Autodesk Inventor part; units mm, degrees
ref_plane "YZ Plane" through (0, 0, 0) normal (1, 0, 0) x (0, 1, 0)
ref_plane "XZ Plane" through (0, 0, 0) normal (0, 1, 0) x (-1, 0, 0)
ref_plane "XY Plane" through (0, 0, 0) normal (0, 0, 1) x (1, 0, 0)
sketch "Skizze1" plane through (0, 0, 0) normal (0, 1, 0) x (-1, 0, 0)
  line L0 (0, 0) -> (17, 0)
  line L1 (17, 0) -> (17, -40)
  line L2 (17, -40) -> (0, -40)
  line L3 (0, -40) -> (0, 0)
  dimension "d0" = 17
  dimension "d1" = 40
extrude "Extrusion1" add sketch "Skizze1" along normal blind 5
sketch "Skizze2" plane through (0, 5, 0) normal (0, 1, 0) x (1, 0, 0)
  line L0 (-17, 0) -> (0, 0)
  line L1 (0, 0) -> (0, 40)
  line L2 (-17, 0) -> (0, 0)
  line L3 (0, 0) -> (0, 10)
  line L4 (0, 10) -> (-17, 10)
  line L5 (-17, 10) -> (-17, 0)
  dimension "d4" = 10
extrude "Extrusion2" add sketch "Skizze2" along normal blind 11
sketch "Skizze3" plane through (0, 16, 0) normal (0, 1, 0) x (1, 0, 0)
  line L0 (-17, 0) -> (0, 0)
  line L1 (0, 0) -> (0, 40)
  line L2 (-17, 0) -> (0, 0)
  line L3 (0, 0) -> (0, 40)
  line L4 (0, 40) -> (-17, 40)
  line L5 (-17, 40) -> (-17, 0)
  dimension "d7" = 17
  dimension "d8" = 40
extrude "Extrusion3" add sketch "Skizze3" along normal blind 5
sketch "Skizze4" plane through (0, 21, 0) normal (0, 1, 0) x (1, 0, 0)
  line L0 (0, 10) -> (0, 40)
  line L1 (0, 40) -> (-8.5, 40)
  line L2 (-8.5, 40) -> (-8.5, 25)
  line L3 (-8.5, 25) -> (0, 25)
  line L4 (0, 25) -> (0, 40)
  circle A0 centre (-8.5, 25) radius 4.5
  point P0 (0, 0)
  dimension "d11" = 8.5
  dimension "d12" = 15
  dimension "d13" = 9
extrude "Extrusion4" cut sketch "Skizze4" against normal blind 21 contours A0 L2 L3 | L3 L2 A0
sketch "Skizze5" plane through (0, 21, 0) normal (0, 1, 0) x (1, 0, 0)
  circle A0 centre (-8.5, 25) radius 4.5
  line L0 (-8.5, 25) -> (0, 25)
  line L1 (0, 0) -> (0, 40)
  line L2 (0, 25) -> (-2, 25)
  line L3 (-2, 25) -> (-3.25, 25)
  line L4 (-3.25, 25) -> (-3.25, 27.55)
  line L5 (-3.25, 27.55) -> (-0.75, 27.55)
  line L6 (-0.75, 27.55) -> (-0.75, 22.45)
  line L7 (-0.75, 22.45) -> (-3.25, 22.45)
  line L8 (-3.25, 22.45) -> (-3.25, 25)
  dimension "d16" = 2
  dimension "d17" = 1.25
  dimension "d18" = 2.55
  dimension "d19" = 2.5
  dimension "d20" = 5.1
extrude "Extrusion5" cut sketch "Skizze5" against normal blind 5 contours L4 L5 L6 L0 | L0 L6 L7 L8
sketch "Skizze6" plane through (0, 5, 0) normal (0, 1, 0) x (1, 0, 0)
  point P0 (0, 0)
sketch "Skizze7" plane through (0, 21, 0) normal (0, 1, 0) x (1, 0, 0)
  point P0 (0, 0)
sketch "Skizze8" plane through (0, 0, 0) normal (1, 0, 0) x (0, 0, -1)
  line L0 (40, 16) -> (40, 21)
  line L1 (40, 20.3408) -> (25, 20.3408)
  line L2 (40, 20.3408) -> (55, 20.3408) construction
  line L3 (25, 20.3408) -> (25, 21)
  line L4 (27.55, 21) -> (22.45, 21)
  line L5 (25, 21) -> (25, 18.5)
  circle A0 centre (25, 18.5) radius 1.5
  point P0 (0, 0)
  dimension "d23" = 15
  dimension "d24" = 180
  dimension "d25" = 2.5
  dimension "d26" = 3
extrude "Extrusion6" cut sketch "Skizze8" against normal blind 10
sketch "Skizze9" plane through (0, 21, 0) normal (0, 1, 0) x (1, 0, 0)
  point P0 (0, 0)
sketch "Skizze10" plane through (0, 21, 0) normal (0, 1, 0) x (1, 0, 0)
  point P0 (0, 0)
sketch "Skizze11" plane through (0, 5, 0) normal (0, 1, 0) x (1, 0, 0)
  point P0 (0, 0)
sketch "Skizze12" plane through (-17, 0, -40) normal (-1, 0, 0) x (0, 0, 1)
  line L0 (40, 21) -> (0, 21)
  line L1 (40, 0) -> (0, 0)
  line L2 (40, 21) -> (30, 21)
  line L3 (30, 0) -> (40, 0)
  line L4 (40, 0) -> (40, 21)
  line L5 (30, 16) -> (0, 16)
  line L6 (30, 21) -> (0, 21)
  line L7 (0, 21) -> (0, 16)
  line L8 (0, 16) -> (30, 16)
  line L9 (30, 5) -> (30, 16)
  line L10 (30, 5) -> (0, 5)
  line L11 (0, 5) -> (0, 0)
  line L12 (0, 0) -> (30, 0)
  line L13 (30, 16) -> (30, 5)
  dimension "d29" = 10
extrude "Extrusion7" add sketch "Skizze12" along normal blind 2.5
sketch "Skizze13" plane through (0, 0, 0) normal (1, 0, 0) x (0, 0, -1)
  line L0 (0, 0) -> (40, 0)
  line L1 (10, 5) -> (40, 5)
  line L2 (40, 0) -> (10, 0)
  line L3 (10, 5) -> (40, 5)
  line L4 (40, 5) -> (40, 0)
  line L5 (0, 0) -> (0, 21)
  line L6 (10, 0) -> (0, 0)
  line L7 (0, 0) -> (0, 21)
  line L8 (0, 21) -> (10, 21)
  line L9 (10, 16) -> (40, 16)
  line L10 (40, 16) -> (10, 16)
  line L11 (10, 21) -> (40, 21)
  line L12 (40, 21) -> (40, 16)
  line L13 (10, 5) -> (10, 16)
  line L14 (10, 5) -> (10, 16)
  circle A0 centre (25, 18.5) radius 1.5
  circle A1 centre (25, 18.5) radius 1.5
  dimension "d32" = 3
extrude "Extrusion8" add sketch "Skizze13" along normal blind 2.5
sketch "Skizze14" plane through (0, 21, 0) normal (0, 1, 0) x (1, 0, 0)
  line L0 (-0.75, 27.55) -> (-3.25, 27.55)
  line L1 (-3.25, 22.45) -> (-3.25, 27.55)
  line L2 (-0.75, 27.55) -> (-3.25, 27.55)
  line L3 (-3.25, 27.55) -> (-3.25, 22.45)
  line L4 (-3.25, 22.45) -> (-0.75, 22.45)
  line L5 (-0.75, 22.45) -> (-0.75, 27.55)
  point P0 (0, 0)
extrude "Extrusion9" add sketch "Skizze14" against normal blind 5
sketch "Skizze15" plane through (0, 21, 0) normal (0, 1, 0) x (1, 0, 0)
  circle A0 centre (-8.5, 25) radius 4.5
  line L0 (-8.5, 25) -> (2.5, 25)
  line L1 (2.5, 26.5) -> (2.5, 23.5)
  line L2 (2.5, 25) -> (-4, 25)
  line L3 (2.5, 25) -> (-0.75, 25)
  line L4 (-0.75, 25) -> (-2, 25)
  line L5 (-2, 25) -> (-2, 22.45)
  line L6 (-2, 22.45) -> (0.5, 22.45)
  line L7 (0.5, 22.45) -> (0.5, 27.55)
  line L8 (0.5, 27.55) -> (-2, 27.55)
  line L9 (0.5, 27.55) -> (3, 27.55) construction
  line L10 (-2, 27.55) -> (-2, 25)
  point P0 (0, 0)
  dimension "d37" = 3.25
  dimension "d38" = 1.25
  dimension "d39" = 2.55
  dimension "d40" = 90
  dimension "d41" = 2.5
  dimension "d42" = 90
  dimension "d43" = 5.1
  dimension "d44" = 90
  dimension "d45" = 2.5
  dimension "d46" = 180
sketch "Skizze16" plane through (0, 21, 0) normal (0, 1, 0) x (1, 0, 0)
  point P0 (0, 0)
extrude "Extrusion10" cut sketch "Skizze15" against normal blind 5 contours L10 L8 L7 L0 | L0 L7 L6 L5
sketch "Skizze17" plane through (2.5, 0, 0) normal (1, 0, 0) x (0, 0, -1)
  circle A0 centre (25, 18.5) radius 1.5
  circle A1 centre (25, 18.5) radius 1.5
  point P0 (0, 0)
  dimension "d49" = 3
sketch "Skizze18" plane through (-3.25, 18.5, -25) normal (-1, 0, 0) x (0, 0, 1)
  circle A0 centre (0, 0) radius 1.5
  point P0 (25, -18.5)
  dimension "d50" = 3
extrude "Extrusion11" cut sketch "Skizze18" against normal blind 8
sketch "Skizze19" plane through (-19.5, 0, 0) normal (0, 0, 1) x (1, 0, 0)
  line L0 (22, 0) -> (0, 0)
  line L1 (0, 21) -> (0, 16)
  line L2 (22, 0) -> (0, 0)
  line L3 (0, 0) -> (0, 21)
  line L4 (0, 21) -> (22, 21)
  line L5 (22, 21) -> (22, 0)
  point P0 (19.5, 0)
extrude "Extrusion12" add sketch "Skizze19" along normal blind 5
sketch "Skizze20" plane through (-19.5, 5, -10) normal (0, 0, -1) x (-1, 0, 0)
  line L0 (0, 11) -> (0, 0)
  line L1 (0, 11) -> (-22, 11)
  line L2 (0, 0) -> (-22, 0)
  line L3 (-22, 0) -> (-22, 11)
  line L4 (-22, 11) -> (0, 11)
  line L5 (0, 11) -> (0, 0)
  point P0 (-19.5, -5)
extrude "Extrusion13" cut sketch "Skizze20" against normal blind 5
sketch "Skizze21" plane through (-19.5, 0, -40) normal (-1, 0, 0) x (0, 0, 1)
  line L0 (0, 0) -> (45, 0)
  line L1 (0, 5) -> (45, 5)
  line L2 (45, 5) -> (45, 0)
  line L3 (45, 0) -> (0, 0)
  line L4 (0, 0) -> (0, 5)
  point P0 (40, 0)
extrude "Extrusion14" add sketch "Skizze21" along normal blind 13.5
sketch "Skizze22" plane through (2.5, 0, 0) normal (1, 0, 0) x (0, 0, -1)
  line L0 (40, 0) -> (-5, 0)
  line L1 (40, 5) -> (5, 5)
  line L2 (-5, 0) -> (40, 0)
  line L3 (40, 0) -> (40, 5)
  line L4 (40, 5) -> (-5, 5)
  line L5 (-5, 5) -> (-5, 0)
  point P0 (0, 0)
extrude "Extrusion15" add sketch "Skizze22" along normal blind 13.5
sketch "Skizze23" plane through (0, 5, 0) normal (0, 1, 0) x (1, 0, 0)
  line L0 (16, 40) -> (10, 40)
  line L1 (10, 40) -> (10, 34)
  line L2 (10, 34) -> (16, 34)
  line L3 (16, 34) -> (16, 40)
  circle A0 centre (10, 34) radius 1.5
  point P0 (0, 0)
  dimension "d61" = 6
  dimension "d62" = 6
  dimension "d63" = 3
extrude "Extrusion16" cut sketch "Skizze23" against normal blind 13.5 contours A0 L2 L1 | L1 L2 A0
sketch "Skizze24" plane through (0, 5, 0) normal (0, 1, 0) x (1, 0, 0)
  line L0 (16, -5) -> (16, 40)
  line L1 (16, -5) -> (10, -5)
  line L2 (10, -5) -> (10, 1)
  line L3 (10, 1) -> (16, 1)
  line L4 (16, 1) -> (16, -5)
  circle A0 centre (10, 1) radius 1.5
  point P0 (0, 0)
  dimension "d66" = 6
  dimension "d67" = 6
  dimension "d68" = 3
extrude "Extrusion17" cut sketch "Skizze24" against normal blind 13.5 contours A0 L2 L3 | L3 L2 A0
sketch "Skizze25" plane through (0, 5, 0) normal (0, 1, 0) x (1, 0, 0)
  line L0 (-33, 40) -> (-33, -5)
  line L1 (-33, 40) -> (-27, 40)
  line L2 (-27, 40) -> (-27, 34)
  line L3 (-27, 34) -> (-33, 34)
  line L4 (-33, 34) -> (-33, 40)
  circle A0 centre (-27, 34) radius 1.5
  point P0 (0, 0)
  dimension "d71" = 6
  dimension "d72" = 6
  dimension "d73" = 3
extrude "Extrusion18" cut sketch "Skizze25" against normal blind 13.5 contours A0 L2 L3 | L3 L2 A0
sketch "Skizze26" plane through (0, 5, 0) normal (0, 1, 0) x (1, 0, 0)
  line L0 (16, -5) -> (-33, -5)
  line L1 (-33, -5) -> (-27, -5)
  line L2 (-27, -5) -> (-27, 1)
  line L3 (-27, 1) -> (-33, 1)
  line L4 (-33, 1) -> (-33, -5)
  circle A0 centre (-27, 1) radius 1.5
  point P0 (0, 0)
  dimension "d76" = 6
  dimension "d77" = 6
  dimension "d78" = 3
extrude "Extrusion19" cut sketch "Skizze26" against normal blind 13.5 contours A0 L3 L2 | L2 L3 A0
sketch "Skizze27" plane through (0, 5, 0) normal (0, 1, 0) x (1, 0, 0)
  line L0 (2.5, -5) -> (16, -5)
  line L1 (16, 40) -> (16, -5)
  line L2 (2.5, -5) -> (16, -5)
  line L3 (16, -5) -> (16, 40)
  line L4 (16, 40) -> (2.5, 40)
  line L5 (2.5, 40) -> (2.5, -5)
  point P0 (0, 0)
extrude "Extrusion20" cut sketch "Skizze27" against normal blind 10
sketch "Skizze28" plane through (0, 5, 0) normal (0, 1, 0) x (1, 0, 0)
  line L0 (-19.5, 5) -> (-19.5, -5)
  line L1 (-33, -5) -> (-33, 40)
  line L2 (-19.5, -5) -> (-33, -5)
  line L3 (-33, -5) -> (-33, 40)
  line L4 (-33, 40) -> (-19.5, 40)
  line L5 (-19.5, 40) -> (-19.5, -5)
  point P0 (0, 0)
extrude "Extrusion21" cut sketch "Skizze28" against normal blind 10
sketch "Skizze29" plane through (0, 0, 0) normal (0, -1, 0) x (1, 0, 0)
  line L0 (2.5, 5) -> (-19.5, 5)
  line L1 (-19.5, -40) -> (-19.5, -5)
  line L2 (2.5, 5) -> (-19.5, 5)
  line L3 (-19.5, 5) -> (-19.5, -40)
  line L4 (-19.5, -40) -> (2.5, -40)
  line L5 (2.5, -40) -> (2.5, 5)
  point P0 (0, 0)
extrude "Extrusion22" add sketch "Skizze29" along normal blind 10
sketch "Skizze30" plane through (0, 5, 0) normal (0, 1, 0) x (1, 0, 0)
  circle A0 centre (-8.5, 25) radius 4.5
  circle A1 centre (-8.5, 25) radius 4.5
  point P0 (0, 0)
  dimension "d87" = 9
extrude "Extrusion23" add sketch "Skizze30" against normal blind 5
extrude "Extrusion24" cut sketch "Skizze30" against normal blind 15
sketch "Skizze31" plane through (2.5, 5, -40) normal (0, 0, -1) x (-1, 0, 0)
  point P0 (2.5, -5)
sketch "Skizze32" plane through (2.5, 0, 0) normal (1, 0, 0) x (0, 0, -1)
  line L0 (-5, -10) -> (-5, 21)
  line L1 (-5, -10) -> (40, -10)
  line L2 (40, -10) -> (40, -5)
  line L3 (40, -5) -> (-5, -5)
  line L4 (-5, -5) -> (-5, -10)
  point P0 (0, 0)
  dimension "d92" = 45
  dimension "d93" = 5
extrude "Extrusion25" add sketch "Skizze32" along normal blind 13.5
sketch "Skizze33" plane through (-19.5, 0, -40) normal (-1, 0, 0) x (0, 0, 1)
  line L0 (45, -10) -> (0, -10)
  line L1 (0, -10) -> (45, -10)
  line L2 (45, -10) -> (45, -5)
  line L3 (45, -5) -> (0, -5)
  line L4 (0, -5) -> (0, -10)
  point P0 (40, 0)
  dimension "d96" = 45
  dimension "d97" = 5
extrude "Extrusion26" add sketch "Skizze33" along normal blind 13.5
sketch "Skizze34" plane through (-19.5, -5, 5) normal (0, 1, 0) x (1, 0, 0)
  line L0 (35.5, 45) -> (-13.5, 45)
  line L1 (-13.5, 45) -> (-7.5, 45)
  line L2 (-7.5, 45) -> (-7.5, 39)
  line L3 (-7.5, 39) -> (-13.5, 39)
  line L4 (-13.5, 39) -> (-13.5, 45)
  circle A0 centre (-7.5, 39) radius 1.5
  point P0 (19.5, 5)
  dimension "d100" = 6
  dimension "d101" = 6
  dimension "d102" = 3
extrude "Extrusion27" cut sketch "Skizze34" against normal blind 5 contours A0 L3 L2 | L2 L3 A0
sketch "Skizze35" plane through (-19.5, -5, 5) normal (0, 1, 0) x (1, 0, 0)
  line L0 (0, 0) -> (-13.5, 0)
  line L1 (-13.5, 0) -> (-7.5, 0)
  line L2 (-7.5, 0) -> (-7.5, 6)
  line L3 (-7.5, 6) -> (-13.5, 6)
  line L4 (-13.5, 6) -> (-13.5, 0)
  circle A0 centre (-7.5, 6) radius 1.5
  point P0 (19.5, 5)
  dimension "d105" = 6
  dimension "d106" = 6
  dimension "d107" = 3
extrude "Extrusion28" cut sketch "Skizze35" against normal blind 5 contours A0 L3 L2 | L2 L3 A0
sketch "Skizze36" plane through (2.5, -5, 5) normal (0, 1, 0) x (1, 0, 0)
  line L0 (13.5, 0) -> (13.5, 45)
  line L1 (13.5, 45) -> (7.5, 45)
  line L2 (7.5, 45) -> (7.5, 39)
  line L3 (7.5, 39) -> (13.5, 39)
  line L4 (13.5, 39) -> (13.5, 45)
  circle A0 centre (7.5, 39) radius 1.5
  point P0 (-2.5, 5)
  dimension "d110" = 6
  dimension "d111" = 6
  dimension "d112" = 3
sketch "Skizze37" plane through (2.5, -5, 5) normal (0, 1, 0) x (1, 0, 0)
  point P0 (-2.5, 5)
extrude "Extrusion29" cut sketch "Skizze36" against normal blind 5 contours A0 L2 L3 | L3 L2 A0
sketch "Skizze38" plane through (2.5, -5, 5) normal (0, 1, 0) x (1, 0, 0)
  line L0 (13.5, 0) -> (13.5, 45)
  line L1 (13.5, 0) -> (7.5, 0)
  line L2 (7.5, 0) -> (7.5, 6)
  line L3 (7.5, 6) -> (13.5, 6)
  line L4 (13.5, 6) -> (13.5, 0)
  circle A0 centre (7.5, 6) radius 1.5
  point P0 (-2.5, 5)
  dimension "d115" = 6
  dimension "d116" = 6
  dimension "d117" = 3
extrude "Extrusion30" cut sketch "Skizze38" against normal blind 5 contours A0 L2 L3 | L3 L2 A0
properties part number "HalterungRillenKugelLager"
Check sheet for the modelled part. Datum: model origin and axes. Units: mm. A direction names the side the tool comes from. Give positions to 0.01 mm unless a question says otherwise; leave off trailing zeros. Write each loop counter-clockwise with the first axis right and the second up, starting at its lowest first coordinate (ties: lowest second). Pieces come first, ordered by that corner, then holes.
Item 1: Cross-section at B-B (x = 10). Enter the section's corners in (y, z), and give its area (3 significant figures).
Item 2: Gauge pin test, flat ends, axial feed: pin 1 (5.5 mm diameter, centred on y = 19, z = -25, fed in from +X); pin 2 (4 mm diameter, centred on y = 15, z = -11.5, fed in from -X); pin 3 (1.5 mm diameter, centred on x = 11, z = -23.5, fed in from +Y). Record the tip position at first contact, or that the pin passes through.
Item 3: Cross-section at D-D (y = 18.5). Enter the section's corners in (x, z), and give its area (3 significant figures).
Item 4: Cross-section at A-A (z = -16.5). Enter the section's corners in (x, y).
Item 5: Cross-section at C-C (z = -1). Enter the section's corners in (x, y).
Item 6: Access from +Z, -Z, +X, -X, +Y, -Y to the whole of each face (thin tool, end or side, straight path). Record for faces 1 (the face through (2.5, 2, -13)), 2 (the face through (1.49, 17.49, -23.89)), 3 (the face through (0.5, 20, -24)), 4 (the face through (-9, 5, -19)).
Item 7: Scan lines: L1, parallel to Z at x = -27, y = -7; L2, parallel to X at y = -6.2, z = -1; L3, parallel to Z at x = -8.5, y = -1. Record each from-to range of solid material in increasing order.
Item 8: Draft check along X on faces 5 (the face through (-1, 19, -22.45)), 6 (the face through (-2, 20, -26)), 7 (the face through (-19.5, 2, -13)), 8 (the face through (-8, -4, -40)). Enter one of: released by +X, released by -X, zero draft, split by the parting line, or undercut.
Report:
1. outline: (-10, -40) - (-5, -40) - (-5, -35.5) - (-10, -35.5) - close; (-10, -32.5) - (-5, -32.5) - (-5, -2.5) - (-10, -2.5) - close; (-10, 0.5) - (-5, 0.5) - (-5, 5) - (-10, 5) - close
1. area: 195 mm2
2. pin 1: stops at x = 2.5
2. pin 2: stops at x = -19.5
2. pin 3: stops at y = -5
3. outline: (-19.5, -40) - (2.5, -40) - (2.5, -26.5) - (0.5, -26.5) - (0.5, -27.55) - (-2, -27.55) - (-2, -26.5) - (-4.26, -26.5) arc R4.5 cw (long way) to (-4.26, -23.5) - (-2, -23.5) - (-2, -22.45) - (0.5, -22.45) - (0.5, -23.5) - (2.5, -23.5) - (2.5, 5) - (-19.5, 5) - close
3. area: 901 mm2
4. outline: (-33, -10) - (16, -10) - (16, -5) - (2.5, -5) - (2.5, 5) - (-19.5, 5) - (-19.5, -5) - (-33, -5) - close; (-19.5, 16) - (2.5, 16) - (2.5, 21) - (-19.5, 21) - close
5. outline: (-33, -10) - (-28.5, -10) - (-28.5, -5) - (-33, -5) - close; (-25.5, -10) - (8.5, -10) - (8.5, -5) - (2.5, -5) - (2.5, 21) - (-19.5, 21) - (-19.5, -5) - (-25.5, -5) - close; (11.5, -10) - (16, -10) - (16, -5) - (11.5, -5) - close
6. face 1: +Z, -Z, +X, +Y
6. face 2: +X
6. face 3: +Y
6. face 4: -Z, +X, -X
7. L1: z = -40 to -35.5, -32.5 to -2.5, 0.5 to 5
7. L2: x = -33 to -28.5, -25.5 to 8.5, 11.5 to 16
7. L3: z = -40 to -29.5, -20.5 to 5
8. face 5: undercut
8. face 6: undercut
8. face 7: released by -X
8. face 8: zero draft
